Drawing for the job (mm, zero at the part's lowest x, y, z). Round coordinates to 2 decimals unless told otherwise and drop trailing zeros. Order: outer loops, then holes, each group sorted by start corner. A loop starts at its lowest first (then second) coordinate and runs counter-clockwise, first axis right, second up. Notation, with made-up numbers: M 51.25,70 L 106.25,70 A30 cw 106.25,94 Z; hole C 20.5,44 d11. An arc over 180 degrees is marked long. One line per item, written item: value. Start each with the question number.
Item 1: Band-saw the part on C-C, the plane z = 51.5. Write the cut outline in (x, y), then the cut area to 3 significant figures.
Item 2: Band-saw the part on A-A, the plane y = 7. Write the cut outline in (x, z), then the cut area to 3 significant figures.
Item 3: Pin check, flat tips, straight feed: pin 1 (5 mm diameter, centred on y = 3, z = 75.5, fed in from -X); pin 2 (5.5 mm diameter, centred on y = 8, z = 126.5, fed in from +X); pin 3 (4 mm diameter, centred on y = 6, z = 132, fed in from -X). Stop position of each tip, or through.
Item 4: Probe L1, parallel to X at y = 7.5, z = 70; L2, parallel to Z at x = 3, y = 11; L3, parallel to X at y = 6.75, z = 131.5. List the from-to ranges inside material, lowest first.
Item 5: Band-saw the part on B-B, the plane z = 122. Write the cut outline in (x, y).
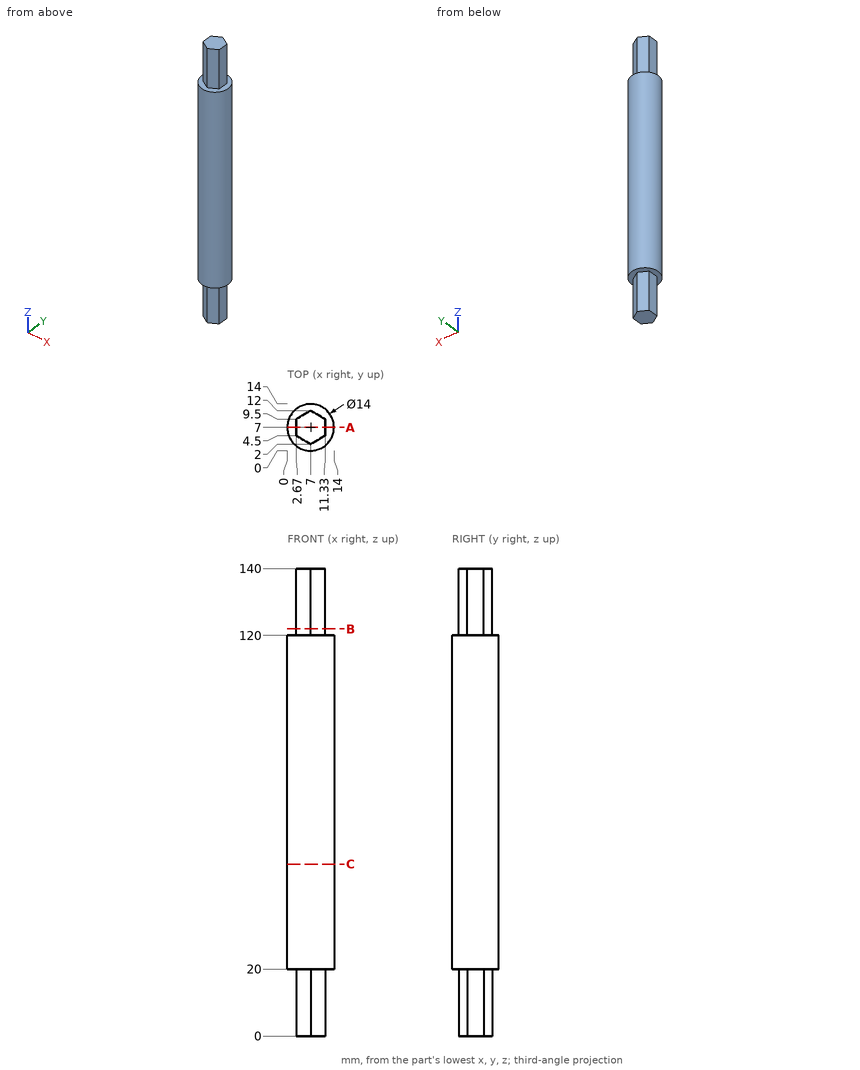
Output:
1. outline: C 7,7 d14
1. area: 154 mm²
2. outline: M 0,20 L 2.67,20 L 2.67,0 L 11.33,0 L 11.33,20 L 14,20 L 14,120 L 11.33,120 L 11.33,140 L 2.67,140 L 2.67,120 L 0,120 Z
2. area: 1,750 mm²
3. pin 1: stops at x = 0.16
3. pin 2: stops at x = 11.33
3. pin 3: stops at x = 2.67
4. L1: x = 0.02 to 13.98
4. L2: z = 20 to 120
4. L3: x = 2.67 to 11.33
5. outline: M 2.67,4.5 L 7,2 L 11.33,4.5 L 11.33,9.5 L 7,12 L 2.67,9.5 Z
